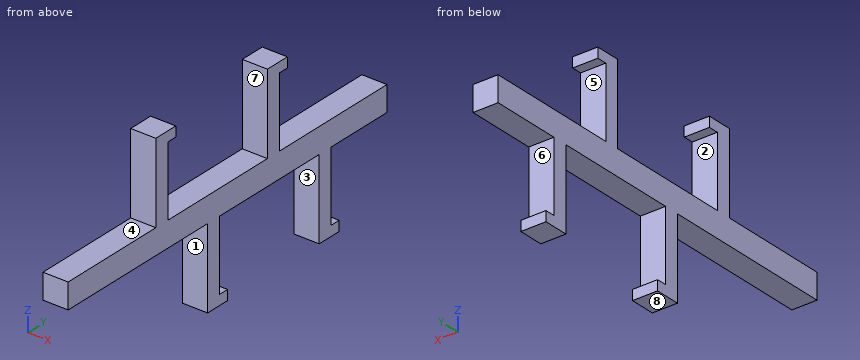
from build123d import *

# Parameters (mm, degrees)
SKETCH1_W           = 6.35
SKETCH1_H           = 6.35
BOSS_EXTRUDE1_DEPTH = 101.6
SKETCH4_W           = 6.35
SKETCH4_H           = 3.81
BOSS_EXTRUDE2_DEPTH = 20.32
SKETCH5_W           = 6.35
SKETCH5_H           = 2.54
BOSS_EXTRUDE3_DEPTH = 2.54
SKETCH6_W           = 6.35
SKETCH6_H           = 3.81
BOSS_EXTRUDE4_DEPTH = 20.32
SKETCH7_W           = 6.35
SKETCH7_H           = 2.54
BOSS_EXTRUDE5_DEPTH = 2.54
SKETCH9_W           = 6.35
SKETCH9_H           = 2.54
BOSS_EXTRUDE6_DEPTH = 2.54
SKETCH8_W           = 6.35
SKETCH8_H           = 2.54
BOSS_EXTRUDE7_DEPTH = 2.54


with BuildPart() as part:
    # Sketch1 → Boss-Extrude1 (new body)
    with BuildSketch(Plane(origin=(0, 0, 0), x_dir=(1, 0, 0), z_dir=(0, 1, 0))):
        Rectangle(SKETCH1_W, SKETCH1_H)
    extrude(amount=BOSS_EXTRUDE1_DEPTH)

    # Sketch4 → Boss-Extrude2 (add)
    with BuildSketch(Plane.XY.offset(3.175)):
        with Locations((0, 29.845)):
            Rectangle(SKETCH4_W, SKETCH4_H)
        with Locations((0, 65.405)):
            Rectangle(SKETCH4_W, SKETCH4_H)
    extrude(amount=BOSS_EXTRUDE2_DEPTH)

    # Sketch5 → Boss-Extrude3 (add)
    with BuildSketch(Plane(origin=(0, 31.75, 0), x_dir=(1, 0, 0), z_dir=(0, 1, 0))):
        with Locations((0, -22.225)):
            Rectangle(SKETCH5_W, SKETCH5_H)
    extrude(amount=BOSS_EXTRUDE3_DEPTH)

    # Sketch6 → Boss-Extrude4 (add)
    with BuildSketch(Plane(origin=(0, 0, -3.175), x_dir=(-1, 0, 0), z_dir=(0, 0, -1))):
        with Locations((0, 81.915)):
            Rectangle(SKETCH6_W, SKETCH6_H)
        with Locations((0, 46.355)):
            Rectangle(SKETCH6_W, SKETCH6_H)
    extrude(amount=BOSS_EXTRUDE4_DEPTH)

    # Sketch7 → Boss-Extrude5 (add)
    with BuildSketch(Plane(origin=(0, 48.26, 0), x_dir=(1, 0, 0), z_dir=(0, 1, 0))):
        with Locations((0, 22.225)):
            Rectangle(SKETCH7_W, SKETCH7_H)
    extrude(amount=BOSS_EXTRUDE5_DEPTH)

    # Sketch9 → Boss-Extrude6 (add)
    with BuildSketch(Plane(origin=(0, 83.82, 0), x_dir=(1, 0, 0), z_dir=(0, 1, 0))):
        with Locations((0, 22.225)):
            Rectangle(SKETCH9_W, SKETCH9_H)
    extrude(amount=BOSS_EXTRUDE6_DEPTH)

    # Sketch8 → Boss-Extrude7 (add)
    with BuildSketch(Plane(origin=(0, 67.31, 0), x_dir=(1, 0, 0), z_dir=(0, 1, 0))):
        with Locations((0, -22.225)):
            Rectangle(SKETCH8_W, SKETCH8_H)
    extrude(amount=BOSS_EXTRUDE7_DEPTH)


solid = part.part
For this review, take the finished solid that the model builds, in its own axes (mm). Face numbers are marked on the shaded views. A direction names the side the tool comes from. Coordinates: 2 decimals unless noted, no trailing zeros. Loops run counter-clockwise (first coordinate to the right, second up) from the corner with the lowest first, then second, coordinate; pieces in that order, holes last. Notation, with made-up numbers: (52.25, 59.5) - (72.25, 59.5) arc R17 cw to (72.25, 86.5) - close; hole circle Ø10 at (54.5, 48.25). An arc over 180 degrees is marked (long way). Use a Markdown table: item, result. Add a question column.
Item 1: For line 1 (Y direction, x = 1.5, z = 10.5); line 2 (Y direction, x = 2.75, z = -14); line 3 (Z direction, x = 1.25, y = 49) (3 decimals), list the stretches that pass through material, from the lowest coordinate up.
Item 2: Insertion check: pin 1 Ø1.3 at (x, y) = (-0.5, 33.5) entering from -Z (3 decimals); pin 2 Ø1.5 at (x, z) = (1, 9) entering from -Y; pin 3 Ø1.3 at (x, y) = (1, 49) entering from +Z (3 decimals). Each pin has a flat end and moves straight along its axis. Give the tip position at first contact, or say it passes through.
Item 3: We need section B-B (x = -1.5). Give the boundary of the cut face in (y, z) (3 decimals).
Item 4: Tool access review of the marked faces 1, 2, 3, 4 and 5: name each direction out of +Z, -Z, +X, -X, +Y, -Y from which nothing blocks a thin tool from reaching the whole face with its end or side.
Item 5: We need section C-C (y = 39.5). Give the boundary of the cut face in (x, z) (3 decimals).
Item 6: We need section A-A (z = -8.5). Give the boundary of the cut face in (x, y) (3 decimals).
Item 7: We need section D-D (y = 29). Give the boundary of the cut face in (x, z) (3 decimals), and give its area (3 significant figures).
Item 8: Mouldability with a two-part tool opening along Z and no side actions: class the marked faces 6, 7 and 8 as pulls with the +Z half, pulls with the -Z half, needs draft (parallel to the pull), parting line crosses it, or undercut.
Results list:
| question | item | result |
|---|---|---|
| 1 | line 1 | y = 27.94 to 31.75, 63.5 to 67.31 |
| 1 | line 2 | y = 44.45 to 48.26, 80.01 to 83.82 |
| 1 | line 3 | z = -23.495 to -20.955, -3.175 to 3.175 |
| 2 | pin 1 | stops at z = -3.175 |
| 2 | pin 2 | stops at y = 27.94 |
| 2 | pin 3 | stops at z = 3.175 |
| 3 | outline | (0, -3.175) - (44.45, -3.175) - (44.45, -23.495) - (50.8, -23.495) - (50.8, -20.955) - (48.26, -20.955) - (48.26, -3.175) - (80.01, -3.175) - (80.01, -23.495) - (86.36, -23.495) - (86.36, -20.955) - (83.82, -20.955) - (83.82, -3.175) - (101.6, -3.175) - (101.6, 3.175) - (67.31, 3.175) - (67.31, 20.955) - (69.85, 20.955) - (69.85, 23.495) - (63.5, 23.495) - (63.5, 3.175) - (31.75, 3.175) - (31.75, 20.955) - (34.29, 20.955) - (34.29, 23.495) - (27.94, 23.495) - (27.94, 3.175) - (0, 3.175) - close |
| 4 | face 1 | -Z, +X, -X, -Y |
| 4 | face 2 | +X, -X |
| 4 | face 3 | -Z, +X, -X |
| 4 | face 4 | +Z, +X, -X, -Y |
| 4 | face 5 | +X, -X, +Y |
| 5 | outline | (-3.175, -3.175) - (3.175, -3.175) - (3.175, 3.175) - (-3.175, 3.175) - close |
| 6 | outline | (-3.175, 44.45) - (3.175, 44.45) - (3.175, 48.26) - (-3.175, 48.26) - close; (-3.175, 80.01) - (3.175, 80.01) - (3.175, 83.82) - (-3.175, 83.82) - close |
| 7 | outline | (-3.175, -3.175) - (3.175, -3.175) - (3.175, 23.495) - (-3.175, 23.495) - close |
| 7 | area | 169 mm^2 |
| 8 | face 6 | undercut |
| 8 | face 7 | needs draft |
| 8 | face 8 | pulls with the -Z half |
